Can you work these out from the model? Positions are in its coordinate system, mm. Face numbers are marked on the shaded views. A direction names the side the tool comes from. Coordinates: 2 decimals unless noted, no trailing zeros. Order: outer loops, then holes, each group sorted by start corner. A loop starts at its lowest first (then second) coordinate and runs counter-clockwise, first axis right, second up. Notation, with made-up numbers: (17, 55.25) -> (26, 55.25) arc R36 cw to (26, 90.25) -> close; hole circle Ø2 at (-2, -9). An arc over 180 degrees is marked (long way). Answer as a JSON object with one key per item and string values. Group by question number.
(1) For pin 1 (0.9 mm diameter, centred on x = -3, z = 1, fed in from +Y); pin 2 (2.5 mm diameter, centred on x = -0.5, z = 2, fed in from -Y); pin 3 (2.5 mm diameter, centred on y = 32, z = -1.6, fed in from +X); pin 4 (1.2 mm diameter, centred on x = 13, y = 0.5, fed in from -Z), each with a flat end and sliding along its axis, tell me the tip position at first contact or that it passes through.
(2) I need wall thicknesses on line 1 (Y direction, x = -12, z = -1.6); line 2 (Y direction, x = -11, z = -0.25); line 3 (Y direction, x = 3.5, z = 2.75). Which ranges of each line are inside material? Lowest first, please.
(3) I want a section at D-D, the plane z = 0.5. List the corners of the cut face in (x, y) for me.
(4) Which directions (+Z, -Z, +X, -X, +Y, -Y) give clear straight access to the entire face, cutting with the end or side of a thin tool? Please do the marked faces 1, 2 and 3.
(5) I want a section at A-A, the plane z = -1.6. State how many separate pieces and enclosed holes the cut face has, plus the area to 3 significant figures.
(6) If we mould it in two halves opening along X, with no side actions, what happens to the marked faces 4, 5 and 6? For each: pulls with the +X half, pulls with the -X half, needs draft (parallel to the pull), parting line crosses it, or undercut.
(7) I want a section at C-C, the plane y = 11. List the corners of the cut face in (x, z) for me, plus the area to 3 significant figures.
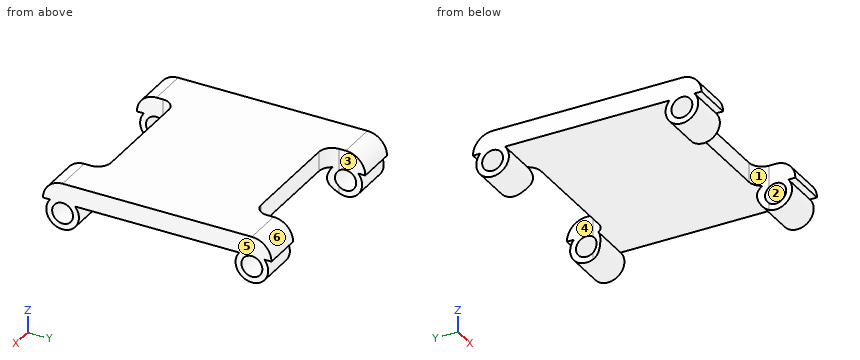
from build123d import *

# Parameters (mm, degrees)
SKETCH1_W                       = 32
SKETCH1_H                       = 35
BOSS_EXTRUDE1_DEPTH             = 3
BOSS_EXTRUDE2_REACH             = 40.601
SKETCH4_R                       = 2.5
SKETCH4_R_2                     = 1.6
BOSS_EXTRUDE2_DIRECTION_2_REACH = 40.601
CUT_EXTRUDE1_DEPTH              = 40.133233958
FILLET1_R                       = 3


with BuildPart() as part:
    # Sketch1 → Boss-Extrude1 (new body)
    with BuildSketch(Plane.XY):
        with Locations((0, 17.5)):
            Rectangle(SKETCH1_W, SKETCH1_H)
    extrude(amount=BOSS_EXTRUDE1_DEPTH)

    # Boss-Extrude2: up to this face of the body (flat: up to its plane)
    boss_extrude2_end = Plane(part.part.faces().sort_by_distance((16, 17.5, 1.5))[0])
    # Sketch4 → Boss-Extrude2 (add, up to the picked face)
    with BuildSketch(Plane(origin=(0, 0, 0), x_dir=(0, 0, -1), z_dir=(1, 0, 0)), mode=Mode.PRIVATE) as boss_extrude2_sk1:
        with Locations((1.6, 32)):
            Circle(SKETCH4_R)
        with Locations(Location((1.6, 32, 0), (0, 0, 180))):
            Circle(SKETCH4_R_2, mode=Mode.SUBTRACT)
    boss_extrude2_tool1 = split(extrude(boss_extrude2_sk1.sketch, amount=BOSS_EXTRUDE2_REACH, mode=Mode.PRIVATE), bisect_by=boss_extrude2_end, keep=Keep.BOTH, mode=Mode.PRIVATE)
    # Sketch4 → Boss-Extrude2 (add, up to the picked face)
    with BuildSketch(Plane(origin=(0, 0, 0), x_dir=(0, 0, -1), z_dir=(1, 0, 0)), mode=Mode.PRIVATE) as boss_extrude2_sk2:
        with Locations((1.6, 3)):
            Circle(SKETCH4_R)
        with Locations(Location((1.6, 3, 0), (0, 0, 180))):
            Circle(SKETCH4_R_2, mode=Mode.SUBTRACT)
    boss_extrude2_tool2 = split(extrude(boss_extrude2_sk2.sketch, amount=BOSS_EXTRUDE2_REACH, mode=Mode.PRIVATE), bisect_by=boss_extrude2_end, keep=Keep.BOTH, mode=Mode.PRIVATE)
    add(boss_extrude2_tool1.solids().sort_by(Axis((0, 32, 0.829289), (1, 0, 0)))[0])
    add(boss_extrude2_tool2.solids().sort_by(Axis((0, 3, 0.829289), (1, 0, 0)))[0])

    # Boss-Extrude2 direction 2: up to this face of the body (flat: up to its plane)
    boss_extrude2_direction_2_end = Plane(part.part.faces().sort_by_distance((-16, 17.5, 1.5))[0])
    # Sketch4 → Boss-Extrude2 direction 2 (add, up to the picked face)
    with BuildSketch(Plane(origin=(0, 0, 0), x_dir=(0, 0, -1), z_dir=(1, 0, 0)), mode=Mode.PRIVATE) as boss_extrude2_direction_2_sk1:
        with Locations((1.6, 32)):
            Circle(SKETCH4_R)
        with Locations(Location((1.6, 32, 0), (0, 0, 180))):
            Circle(SKETCH4_R_2, mode=Mode.SUBTRACT)
    boss_extrude2_direction_2_tool1 = split(extrude(boss_extrude2_direction_2_sk1.sketch, amount=-BOSS_EXTRUDE2_DIRECTION_2_REACH, mode=Mode.PRIVATE), bisect_by=boss_extrude2_direction_2_end, keep=Keep.BOTH, mode=Mode.PRIVATE)
    # Sketch4 → Boss-Extrude2 direction 2 (add, up to the picked face)
    with BuildSketch(Plane(origin=(0, 0, 0), x_dir=(0, 0, -1), z_dir=(1, 0, 0)), mode=Mode.PRIVATE) as boss_extrude2_direction_2_sk2:
        with Locations((1.6, 3)):
            Circle(SKETCH4_R)
        with Locations(Location((1.6, 3, 0), (0, 0, 180))):
            Circle(SKETCH4_R_2, mode=Mode.SUBTRACT)
    boss_extrude2_direction_2_tool2 = split(extrude(boss_extrude2_direction_2_sk2.sketch, amount=-BOSS_EXTRUDE2_DIRECTION_2_REACH, mode=Mode.PRIVATE), bisect_by=boss_extrude2_direction_2_end, keep=Keep.BOTH, mode=Mode.PRIVATE)
    add(boss_extrude2_direction_2_tool1.solids().sort_by(Axis((0, 32, 0.829289), (-1, 0, 0)))[0])
    add(boss_extrude2_direction_2_tool2.solids().sort_by(Axis((0, 3, 0.829289), (-1, 0, 0)))[0])

    # Sketch5 → Cut-Extrude1 (cut, through all)
    with BuildSketch(Plane.XY.offset(3)):
        with BuildLine():
            Line((-10, 35), (-10, 31))
            ThreePointArc((-10, 31), (-9.414213562, 29.585786438), (-8, 29))
            Line((-8, 29), (8, 29))
            ThreePointArc((8, 29), (9.414213562, 29.585786438), (10, 31))
            Line((10, 31), (10, 35))
            Line((10, 35), (-10, 35))
        make_face()
        with BuildLine():
            Line((-10, 0), (-10, 4))
            ThreePointArc((-10, 4), (-9.414213562, 5.414213562), (-8, 6))
            Line((-8, 6), (8, 6))
            ThreePointArc((8, 6), (9.414213562, 5.414213562), (10, 4))
            Line((10, 4), (10, 0))
            Line((10, 0), (-10, 0))
        make_face()
    extrude(amount=-CUT_EXTRUDE1_DEPTH, mode=Mode.SUBTRACT)

    # Fillet1
    fillet1_edges = [part.edges().sort_by_distance(p)[0] for p in [
        (13, 0, 3),
        (-13, 0, 3),
        (13, 35, 3),
        (-13, 35, 3),
    ]]
    fillet(fillet1_edges, radius=FILLET1_R - 0.0001)  # a hair under: the kernel refuses the full size


solid = part.part
Computed values:
{
 "1": {"pin 1": "stops at y = 29", "pin 2": "stops at y = 6", "pin 3": "passes through", "pin 4": "stops at z = -3.22"},
 "2": {"line 1": "y = 0.5 to 1.4, 4.6 to 5.5, 29.5 to 30.4, 33.6 to 34.5", "line 2": "y = 0.9 to 2.14, 3.86 to 5.1, 29.9 to 31.14, 32.86 to 34.1", "line 3": "y = 6 to 29"},
 "3": {"outline": "(-16, 0.04) -> (-10, 0.04) -> (-10, 4) arc R2 cw to (-8, 6) -> (8, 6) arc R2 cw to (10, 4) -> (10, 0.04) -> (16, 0.04) -> (16, 34.96) -> (10, 34.96) -> (10, 31) arc R2 cw to (8, 29) -> (-8, 29) arc R2 cw to (-10, 31) -> (-10, 34.96) -> (-16, 34.96) -> close"},
 "4": {"face 1": "+Z, -Z, -Y", "face 2": "+X, -X", "face 3": "+Z, -Z, +Y"},
 "5": {"separate pieces": "8", "enclosed holes": "0", "area": "44.4 mm2"},
 "6": {"face 4": "undercut", "face 5": "pulls with the +X half", "face 6": "needs draft"},
 "7": {"outline": "(-16, 0) -> (16, 0) -> (16, 3) -> (-16, 3) -> close", "area": "96.0 mm2"}
}
